from build123d import *

# Parameters (mm, degrees)
F0_W          = 100
F0_H          = 40
F1_DEPTH      = 10
F4_DEPTH      = 10
F5_W          = 40
F5_H          = 3
F6_DEPTH      = 40.001
F7_R          = 2.25
F8_DEPTH      = 40.001
F9_R          = 4.5
F10_DEPTH     = 5.7
F11_T1_DEPTH  = 40
F11_T3_DEPTH  = 40
F11_T5_DEPTH  = 50
F11_T7_DEPTH  = 50
F11_T9_DEPTH  = 50
F11_T11_DEPTH = 50
F12_R         = 3


# Not quite as in the source:
# - a fillet or chamfer that OpenCascade refuses, or shapes differently, is made with other operations: its cross-section is extruded or revolved along the edge and cut away or added


with BuildPart() as f1:
    # F0 (on Top) → F1 (new body)
    with BuildSketch(Plane.XY):
        with Locations((50, 20)):
            Rectangle(F0_W, F0_H)
    extrude(amount=F1_DEPTH)

    # F3 (on face) → F4 (join)
    with BuildSketch(Plane(origin=(0, 40, 0), x_dir=(-1, 0, 0), z_dir=(0, 1, 0))):
        with BuildLine():
            Line((-70, 35), (-70, 0))
            Line((-70, 0), (-30, 0))
            Line((-30, 0), (-30, 35))
            ThreePointArc((-30, 35), (-50, 55), (-70, 35))
        make_face()
    extrude(amount=-F4_DEPTH)

    # F5 (on face) → F6 (cut, through all)
    with BuildSketch(Plane(origin=(0, 40, 0), x_dir=(-1, 0, 0), z_dir=(0, 1, 0))):
        with Locations((-50, 1.5)):
            Rectangle(F5_W, F5_H)
    extrude(amount=-F6_DEPTH, mode=Mode.SUBTRACT)

    # F7 (on face) → F8 (cut, through all)
    with BuildSketch(Plane(origin=(0, 40, 0), x_dir=(-1, 0, 0), z_dir=(0, 1, 0))):
        with Locations((-50, 35)):
            Circle(F7_R)
    extrude(amount=-F8_DEPTH, mode=Mode.SUBTRACT)

    # F9 (on face) → F10 (cut)
    with BuildSketch(Plane(origin=(0, 40, 0), x_dir=(-1, 0, 0), z_dir=(0, 1, 0))):
        with Locations((-50, 35)):
            Circle(F9_R)
    extrude(amount=-F10_DEPTH, mode=Mode.SUBTRACT)

    # F11: fillet of radius 8 on 6 edges, made by hand

    # F11_s2 → F11_t1 (join)
    with BuildSketch(Plane.XZ.offset(-40)):
        with BuildLine():
            ThreePointArc((70, 0), (67.2191036167, 2.2111025509), (63.7550020016, 3))
            Line((63.7550020016, 3), (70, 3))
            Line((70, 3), (70, 0))
        make_face()
    extrude(amount=F11_T1_DEPTH)

    # F11_s4 → F11_t3 (join)
    with BuildSketch(Plane.XZ.offset(-40)):
        with BuildLine():
            ThreePointArc((36.2449979984, 3), (32.7808963833, 2.2111025509), (30, 0))
            Line((30, 0), (30, 3))
            Line((30, 3), (36.2449979984, 3))
        make_face()
    extrude(amount=F11_T3_DEPTH)

    # F11_s6 → F11_t5 (cut)
    with BuildSketch(Plane.XY.offset(-20)):
        with BuildLine():
            ThreePointArc((0, 32), (2.3431457505, 37.6568542495), (8, 40))
            Line((8, 40), (0, 40))
            Line((0, 40), (0, 32))
        make_face()
    extrude(amount=F11_T5_DEPTH, mode=Mode.SUBTRACT)

    # F11_s8 → F11_t7 (cut)
    with BuildSketch(Plane.XY.offset(-20)):
        with BuildLine():
            ThreePointArc((0, 8), (2.3431457505, 2.3431457505), (8, 0))
            Line((8, 0), (0, 0))
            Line((0, 0), (0, 8))
        make_face()
    extrude(amount=F11_T7_DEPTH, mode=Mode.SUBTRACT)

    # F11_s10 → F11_t9 (cut)
    with BuildSketch(Plane.XY.offset(-20)):
        with BuildLine():
            ThreePointArc((92, 40), (97.6568542495, 37.6568542495), (100, 32))
            Line((100, 32), (100, 40))
            Line((100, 40), (92, 40))
        make_face()
    extrude(amount=F11_T9_DEPTH, mode=Mode.SUBTRACT)

    # F11_s12 → F11_t11 (cut)
    with BuildSketch(Plane.XY.offset(-20)):
        with BuildLine():
            ThreePointArc((92, 0), (97.6568542495, 2.3431457505), (100, 8))
            Line((100, 8), (100, 0))
            Line((100, 0), (92, 0))
        make_face()
    extrude(amount=F11_T11_DEPTH, mode=Mode.SUBTRACT)

    # F12
    f12_edges = [f1.edges().sort_by_distance(p)[0] for p in [
        (50, 40, 55),
        (50, 30, 55),
        (30, 40, 22.5),
        (70, 40, 22.5),
        (30, 30, 22.5),
        (70, 30, 22.5),
    ]]
    fillet(f12_edges, radius=F12_R)


solid = f1.part
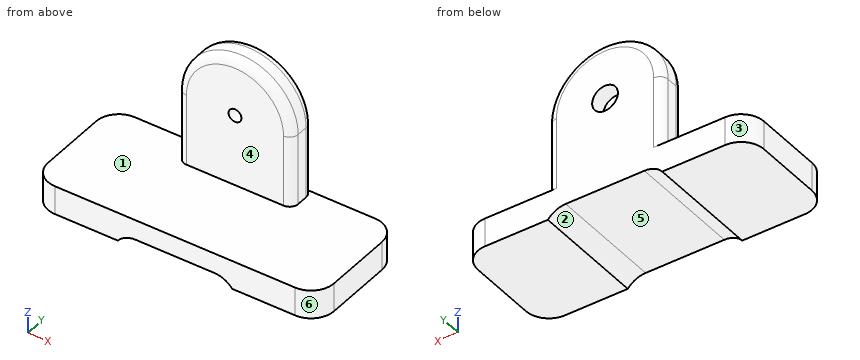
Read the model definition and answer for the solid it produces. Units are mm, in the model's axes. Face numbers are marked on the shaded views. A direction names the side the tool comes from. Round coordinates to 2 decimals unless told otherwise and drop trailing zeros. Loops run counter-clockwise (first coordinate to the right, second up) from the corner with the lowest first, then second, coordinate; pieces in that order, holes last.
Q1. Section B-B on y = 16 is taken. Write down the section's boundary in (x, z) (3 decimals).
Q2. Determine the mould class of the marked faces 1, 2 and 3 for opening direction X: released by +X, released by -X, zero draft, split by the parting line, or undercut.
Q3. Which of the six approach directions +Z, -Z, +X, -X, +Y, -Y give full straight-line access (tool end or side, diameter ignored) to the marked faces 4, 5 and 6?
Q4. Each of these flat-tipped pins is pushed along its axis until it touches: pin 1 (5.5 mm diameter, centred on x = 50, z = 35, fed in from -Y); pin 2 (6 mm diameter, centred on y = 32.5, z = 14, fed in from -X); pin 3 (10 mm diameter, centred on x = 35.5, y = 5, fed in from -Z). Where does it stop, or does it pass through?
Q5. Consider probe 1 along Z at (x, y) = (50, 36.9); probe 2 along Z at (x, y) = (92.5, 27.5); probe 3 along Z at (x, y) = (43.5, 28). Determine where each line is inside the solid, lowest interval first.
Q6. Section A-A on x = 50 is taken. Write down the section's boundary in (y, z), and give its area (3 significant figures).
Q7. Section C-C on x = 23.5 is taken. Write down the section's boundary in (y, z).
Output:
1. outline: (0, 0) - (30, 0) arc R8 cw to (36.245, 3) - (63.755, 3) arc R8 cw to (70, 0) - (100, 0) - (100, 10) - (0, 10) - close
2. face 1: zero draft
2. face 2: undercut
2. face 3: released by -X
3. face 4: +Z, +X, -X, -Y
3. face 5: -Z, +Y, -Y
3. face 6: +Z, -Z, +X, -Y
4. pin 1: stops at y = 30
4. pin 2: stops at x = 30
4. pin 3: stops at z = 0.57
5. probe 1: z = 3 to 30.5, 39.5 to 55
5. probe 2: z = 0 to 10
5. probe 3: z = 3 to 10
6. outline: (0, 3) - (40, 3) - (40, 30.5) - (34.3, 30.5) - (34.3, 32.75) - (30, 32.75) - (30, 10) - (0, 10) - close; (30, 37.25) - (34.3, 37.25) - (34.3, 39.5) - (40, 39.5) - (40, 52) arc R3 ccw to (37, 55) - (33, 55) arc R3 ccw to (30, 52) - close
6. area: 655 mm2
7. outline: (0, 0) - (40, 0) - (40, 10) - (0, 10) - close
